For this review, take the finished solid that the model builds, in its own axes (mm). Give positions to 0.01 mm unless a question says otherwise; leave off trailing zeros. Loops run counter-clockwise (first coordinate to the right, second up) from the corner with the lowest first, then second, coordinate; pieces in that order, holes last. Notation, with made-up numbers: (-18, -18) -> (9, -18) arc R17 ccw to (9, 0) -> close; hole circle Ø8 at (54, 7). An arc over 180 degrees is marked (long way). Write each question's results on one line, items separated by ' | '. Start each with the question number.
```python
from build123d import *

# Parameters (mm, degrees)
SKETCH2_W           = 78
SKETCH2_H           = 10
BOSS_EXTRUDE1_DEPTH = 3.175
SKETCH3_R           = 2.5
CUT_EXTRUDE1_DEPTH  = 3.175
CUT_EXTRUDE2_REACH  = 41.447
SKETCH4_R           = 1
FILLET1_R           = 2


with BuildPart() as part:
    # Sketch2 → Boss-Extrude1 (new body)
    with BuildSketch(Plane(origin=(0, 0, 0), x_dir=(1, 0, 0), z_dir=(0, 1, 0))):
        Rectangle(SKETCH2_W, SKETCH2_H)
    extrude(amount=BOSS_EXTRUDE1_DEPTH)

    # Sketch3 → Cut-Extrude1 (cut)
    with BuildSketch(Plane(origin=(0, 3.175, 0), x_dir=(1, 0, 0), z_dir=(0, 1, 0))):
        with Locations(Location((-34, 0, 0), (0, 0, 270))):
            Circle(SKETCH3_R)
        with Locations(Location((34, 0, 0), (0, 0, 90))):
            Circle(SKETCH3_R)
    extrude(amount=-CUT_EXTRUDE1_DEPTH, mode=Mode.SUBTRACT)

    # Sketch4 → Cut-Extrude2 (cut, up to next)
    with BuildSketch(Plane(origin=(0, 3.175, 0), x_dir=(1, 0, 0), z_dir=(0, 1, 0)), mode=Mode.PRIVATE) as cut_extrude2_sk1:
        with Locations(Location((-19.5, 0, 0), (0, 0, 270))):
            Circle(SKETCH4_R)
    cut_extrude2_tool1 = extrude(cut_extrude2_sk1.sketch, amount=-CUT_EXTRUDE2_REACH, mode=Mode.PRIVATE) & part.part
    add(cut_extrude2_tool1.solids().sort_by_distance((-19.5, 3.175, 0))[0], mode=Mode.SUBTRACT)

    # Fillet1
    fillet1_edges = [part.edges().sort_by_distance(p)[0] for p in [
        (39, 1.5875, 5),
        (-39, 1.5875, 5),
        (-39, 1.5875, -5),
        (39, 1.5875, -5),
    ]]
    fillet(fillet1_edges, radius=FILLET1_R)


solid = part.part
```
1. We need section C-C (y = 1.25). Write out the cut boundary in (x, z).
2. Wall thickness on L1, parallel to X at y = 2.45, z = 0; L2, parallel to X at y = 0.75, z = 1.5; L3, parallel to X at y = 0.4, z = -0.5: over which ranges is each line inside the solid? List them lowest first.
3. For pin 1 Ø4 at (x, z) = (-24, 0) entering from -Y; pin 2 Ø1.8 at (x, z) = (-19.5, 0) entering from +Y, all flat-tipped, find the tip position at first contact; note any pin that passes through.
4. We need section A-A (z = 0). Write out the cut boundary in (x, y) (3 decimals).
5. We need section D-D (x = 34). Write out the cut boundary in (y, z) (3 decimals), plus the area to 3 significant figures.
6. Draft analysis for pull direction X (two halves, no side actions). For faces 1 (the flat face through (-1, 2, 5)), 2 (the cylindrical face through (-38.43, 1.61, 4.4)), 3 (the cylindrical face through (-20.476, 1.61, -0.217)), state which applies: released by +X, released by -X, zero draft, split by the parting line, or undercut.
7. We need section B-B (x = -19.5). Write out the cut boundary in (y, z) (3 decimals).
Response:
1) outline: (-39, -3) arc R2 ccw to (-37, -5) -> (37, -5) arc R2 ccw to (39, -3) -> (39, 3) arc R2 ccw to (37, 5) -> (-37, 5) arc R2 ccw to (-39, 3) -> close; hole circle Ø5 at (-34, 0); hole circle Ø2 at (-19.5, 0); hole circle Ø5 at (34, 0)
2) L1: x = -39 to -36.5, -31.5 to -20.5, -18.5 to 31.5, 36.5 to 39 | L2: x = -39 to -36, -32 to 32, 36 to 39 | L3: x = -39 to -36.45, -31.55 to -20.37, -18.63 to 31.55, 36.45 to 39
3) pin 1: stops at y = 0 | pin 2: passes through
4) outline: (-39, 0) -> (-36.5, 0) -> (-36.5, 3.175) -> (-39, 3.175) -> close; (-31.5, 0) -> (-20.5, 0) -> (-20.5, 3.175) -> (-31.5, 3.175) -> close; (-18.5, 0) -> (31.5, 0) -> (31.5, 3.175) -> (-18.5, 3.175) -> close; (36.5, 0) -> (39, 0) -> (39, 3.175) -> (36.5, 3.175) -> close
5) outline: (0, -5) -> (3.175, -5) -> (3.175, -2.5) -> (0, -2.5) -> close; (0, 2.5) -> (3.175, 2.5) -> (3.175, 5) -> (0, 5) -> close | area: 15.9 mm2
6) face 1: zero draft | face 2: released by -X | face 3: undercut
7) outline: (0, -5) -> (3.175, -5) -> (3.175, -1) -> (0, -1) -> close; (0, 1) -> (3.175, 1) -> (3.175, 5) -> (0, 5) -> close
